Design review of the part shown in the three views and the two pictorial views. Dimensions are in mm from the part's minimum x, y and z. A direction names the side the tool comes from. Round coordinates to 2 decimals unless told otherwise and drop trailing zeros. Write each loop counter-clockwise with the first axis right and the second up, starting at its lowest first coordinate (ties: lowest second). Pieces come first, ordered by that corner, then holes. Notation, with made-up numbers: (69, 69) -> (95, 69) arc R8 ccw to (95, 82) -> close; hole circle Ø7 at (-26, 10.5). An arc over 180 degrees is marked (long way). Return JSON: item names as keys, results as strings. Group by question number.
1. Mouldability with a two-part tool opening along Y and no side actions: class the marked faces 3, 4 and 5 as pulls with the +Y half, pulls with the -Y half, needs draft (parallel to the pull), parting line crosses it, or undercut.
2. Tool access review of the marked faces 1 and 2: name each direction out of +Z, -Z, +X, -X, +Y, -Y from which nothing blocks a thin tool from reaching the whole face with its end or side.
3. Take a section at D-D, the plane y = 5. Write out the cut boundary in (x, z), then the cut area to 4 significant figures.
4. Take a section at C-C, the plane z = 2. Write out the cut boundary in (x, y), then the cut area to 3 significant figures.
5. Take a section at A-A, the plane x = 3.5. Write out the cut boundary in (y, z), then the cut area to 3 significant figures.
6. For line 1 along Z through (x, y) = (8.5, 4.5); line 2 along X through (y, z) = (1.75, 4); line 3 along Y through (x, z) = (5, 15.5), list the stretches that pass through material, from the lowest coordinate up. Write a range as from..to.
7. Take a section at B-B, the plane y = 7. Write out the cut boundary in (x, z).
8. Clearance check with flat-ended pins moving along their axes: P1, Ø6, axis at x = 2.5, z = 8, coming from the -Y side; P2, Ø4, axis at y = 5, z = 2.75, coming from the -X side; P3, Ø3, axis at x = 10, y = 6, coming from the -Z side; P4, Ø4, axis at x = 5, y = 5, coming from the +Z side. State where each tip first meets the part, or that it passes through.
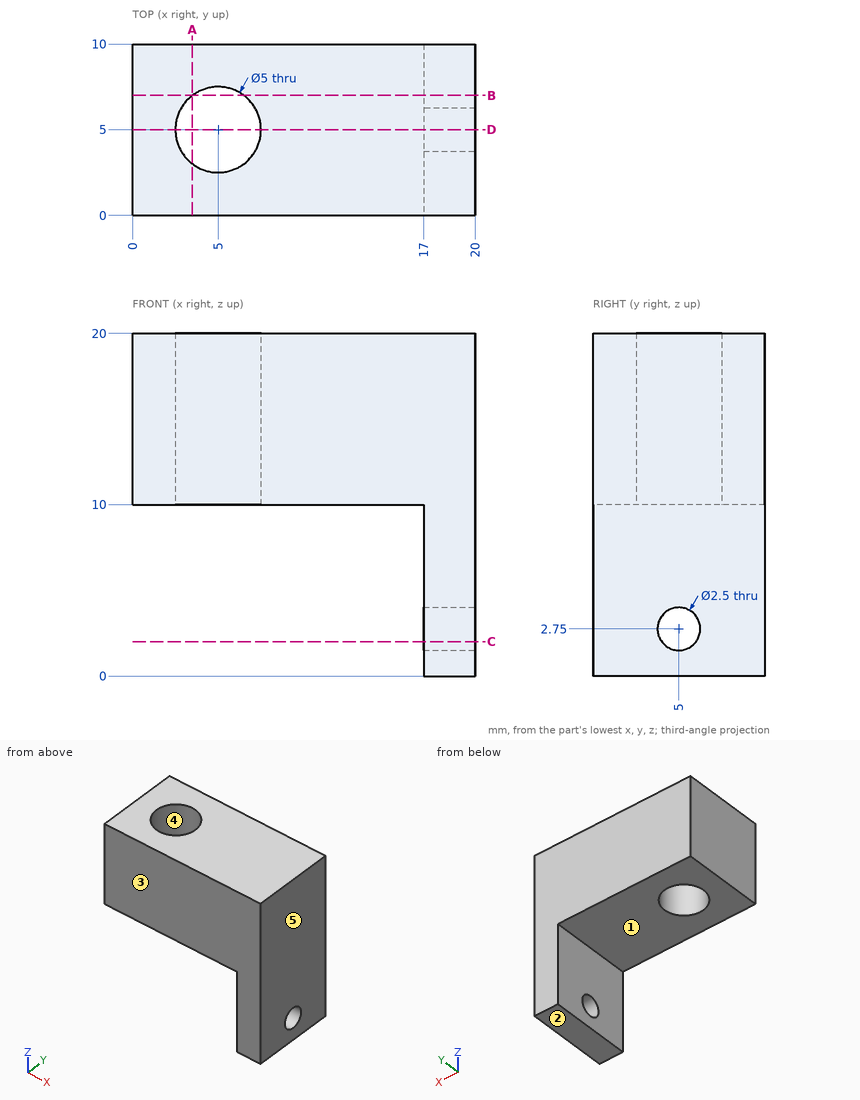
Output:
{
 "1": {"face 3": "pulls with the -Y half", "face 4": "undercut", "face 5": "needs draft"},
 "2": {"face 1": "-Z, -X, +Y, -Y", "face 2": "-Z, +X, -X, +Y, -Y"},
 "3": {"outline": "(0, 10) -> (2.5, 10) -> (2.5, 20) -> (0, 20) -> close; (7.5, 10) -> (17, 10) -> (17, 4) -> (20, 4) -> (20, 20) -> (7.5, 20) -> close; (17, 0) -> (20, 0) -> (20, 1.5) -> (17, 1.5) -> close", "area": "172.5 mm^2"},
 "4": {"outline": "(17, 0) -> (20, 0) -> (20, 4) -> (17, 4) -> close; (17, 6) -> (20, 6) -> (20, 10) -> (17, 10) -> close", "area": "24.0 mm^2"},
 "5": {"outline": "(0, 10) -> (3, 10) -> (3, 20) -> (0, 20) -> close; (7, 10) -> (10, 10) -> (10, 20) -> (7, 20) -> close", "area": "60.0 mm^2"},
 "6": {"line 1": "z = 10..20", "line 2": "x = 17..20", "line 3": "y = 0..2.5, 7.5..10"},
 "7": {"outline": "(0, 10) -> (3.5, 10) -> (3.5, 20) -> (0, 20) -> close; (6.5, 10) -> (17, 10) -> (17, 0) -> (20, 0) -> (20, 20) -> (6.5, 20) -> close"},
 "8": {"P1": "stops at y = 0", "P2": "stops at x = 17", "P3": "stops at z = 10", "P4": "passes through"}
}
